```python
from build123d import *

# Parameters (mm, degrees)
SKETCH2_R           = 2.65
BOSS_EXTRUDE1_DEPTH = 10
SKETCH5_R           = 2.5
CHAMFER1_SIZE       = 3
FILLET4_R           = 4
SKETCH9_R           = 6
SKETCH9_R_2         = 2.2
BOSS_EXTRUDE2_DEPTH = 4
LPATTERN1_COUNT     = 2
LPATTERN1_PITCH     = 30
CHAMFER2_SIZE       = 4


with BuildPart() as part:
    # Sketch2 → Boss-Extrude1 (new, symmetric)
    with BuildSketch(Plane.XY):
        with BuildLine():
            ThreePointArc((-73.989796594, 16), (-75.457580373, 6.053392794), (-75.594245813, -4))
            Line((-75.594245813, -4), (-51.34428877, -4))
            ThreePointArc((-51.34428877, -4), (-42.918193786, -7.205281597), (-37.5, 0))
            Line((-37.5, 0), (-21.763957799, 0))
            Line((-21.763957799, 0), (-5.763957799, 16))
            Line((-5.763957799, 16), (-73.989796594, 16))
        make_face()
        with Locations((-45, 0)):
            Circle(SKETCH2_R, mode=Mode.SUBTRACT)
    extrude(amount=BOSS_EXTRUDE1_DEPTH, both=True)

    # Sketch3 → Cut-Revolve1 (revolve, cut)
    with BuildSketch(Plane.XY, mode=Mode.PRIVATE) as cut_revolve1_sk:
        Polygon((-76.457580373, 8), (-75.457580373, 8), (-50.457580373, 8), (-50.457580373, 12.2), (-70.457580373, 12.2), (-76.457580373, 12.2), align=None)
        Polygon((-76.457580373, 15.2), (-76.457580373, 12.2), (-70.457580373, 12.2), align=None)
    revolve(cut_revolve1_sk.sketch.rotate(Axis((-75.457580373, 8, 0), (1, 0, 0)), 90), axis=Axis((-75.457580373, 8, 0), (1, 0, 0)), mode=Mode.SUBTRACT)

    # Cut-Sweep2: sweep along a path in Sketch7
    with BuildLine(Plane.XY) as cut_sweep2_path:
        Line((-50.457580373, 8), (-25.763957799, 8))
        ThreePointArc((-25.763957799, 8), (-22.228423893, 9.464466094), (-20.763957799, 13))
        Line((-20.763957799, 13), (-20.763957799, 16))
    # Sketch5 → Cut-Sweep2 (sweep, cut)
    with BuildSketch(Plane(origin=(0, 16, 0), x_dir=(1, 0, 0), z_dir=(0, 1, 0))):
        with Locations((-20.763957799, 0)):
            Circle(SKETCH5_R)
    sweep(path=cut_sweep2_path.line, mode=Mode.SUBTRACT)

    # Chamfer1
    # the kernel refuses this chamfer: 3 mm, written as the material it takes off along each edge
    with BuildSketch(Plane(origin=(-50.457580373, 8, 0), x_dir=(0, -1, 0), z_dir=(0, 0, 1))) as chamfer1_piece_1_section:
        Polygon((2.5 + CHAMFER1_SIZE, 0), (2.5, CHAMFER1_SIZE), (2.5, 0), align=None)
    chamfer1_piece_1 = revolve(axis=Axis((-50.457580373, 8, 0), (1, 0, 0)), mode=Mode.PRIVATE)
    chamfer1_piece_1 = chamfer1_piece_1 & Plane(origin=(-48.295596493, 8, 0), x_dir=(0, 0, 1), z_dir=(-1, 0, 0)) * Cylinder(4.2, 22, mode=Mode.PRIVATE)
    add(chamfer1_piece_1, mode=Mode.SUBTRACT)

    # Fillet4
    fillet4_edges = [part.edges().sort_by_distance(p)[0] for p in [
        (-21.763957799, 0, 0),
        (-37.5, 0, 0),
        (-51.34428877, -4, 0),
    ]]
    fillet(fillet4_edges, radius=FILLET4_R)

    # Sketch9 → Boss-Extrude2 (add)
    # profile 1 of 3: a face of its own
    with BuildSketch(Plane(origin=(0, 16, 0), x_dir=(1, 0, 0), z_dir=(0, 1, 0))):
        with Locations((-53.989796594, 16)):
            Circle(SKETCH9_R)
        with Locations(Location((-53.989796594, 16, 0), (0, 0, 270))):
            Circle(SKETCH9_R_2, mode=Mode.SUBTRACT)
    # profile 2 of 3: a face of its own
    with BuildSketch(Plane(origin=(0, 16, 0), x_dir=(1, 0, 0), z_dir=(0, 1, 0))):
        with BuildLine():
            ThreePointArc((-47.989796594, 16), (-49.747155907, 11.757359313), (-53.989796594, 10))
            Line((-53.989796594, 10), (-43.989796594, 10))
            Line((-43.989796594, 10), (-48.695678947, 18.823529412))
            ThreePointArc((-48.695678947, 18.823529412), (-48.168941593, 17.45521375), (-47.989796594, 16))
        make_face()
    # profile 3 of 3: a face of its own
    with BuildSketch(Plane(origin=(0, 16, 0), x_dir=(1, 0, 0), z_dir=(0, 1, 0))):
        with BuildLine():
            Line((-59.283914241, 18.823529412), (-63.989796594, 10))
            Line((-63.989796594, 10), (-53.989796594, 10))
            ThreePointArc((-53.989796594, 10), (-59.134754148, 12.913025467), (-59.283914241, 18.823529412))
        make_face()
    boss_extrude2 = extrude(amount=-BOSS_EXTRUDE2_DEPTH)

    # LPattern1: Boss-Extrude2 ×2
    with Locations(*[(i * LPATTERN1_PITCH, 0, 0) for i in range(1, LPATTERN1_COUNT)]):
        add(boss_extrude2)

    # Chamfer2
    # the kernel refuses this chamfer: 4 mm, written as the material it adds along each edge
    with BuildSketch(Plane(origin=(-33.703064642, 12, -10), x_dir=(0, -0.9996219169112968, 0.027495876610586494), z_dir=(-1, 0, 0))) as chamfer2_piece_1_section:
        Polygon((CHAMFER2_SIZE * 0.999621916911, -CHAMFER2_SIZE * 0.0274958766106), (-CHAMFER2_SIZE * 0.0274958766106, -CHAMFER2_SIZE * 0.999621916911), (0, 0), align=None)
    chamfer2_piece_1 = extrude(amount=40.573463904, mode=Mode.PRIVATE)
    chamfer2_piece_1 = split(chamfer2_piece_1, bisect_by=Plane(origin=(-33.908180605, 9.955648468, -10.153029979), z_dir=(0.882352941176471, 0, 0.4705882352941171)), keep=Keep.TOP, mode=Mode.PRIVATE)
    add(chamfer2_piece_1)
    with BuildSketch(Plane(origin=(-33.703064642, 12, -10), x_dir=(0, -0.9996219169112968, 0.027495876610586494), z_dir=(-1, 0, 0))) as chamfer2_piece_2_section:
        Polygon((CHAMFER2_SIZE * 0.999621916911, -CHAMFER2_SIZE * 0.0274958766106), (-CHAMFER2_SIZE * 0.0274958766106, -CHAMFER2_SIZE * 0.999621916911), (0, 0), align=None)
    chamfer2_piece_2 = extrude(amount=40.573463904, mode=Mode.PRIVATE)
    chamfer2_piece_2 = split(chamfer2_piece_2, bisect_by=Plane(origin=(-61.252355545, 10.648848957, -15.132701966), z_dir=(0.882352941176471, 0, 0.4705882352941171)), keep=Keep.TOP, mode=Mode.PRIVATE)
    chamfer2_piece_2 = split(chamfer2_piece_2, bisect_by=Plane(origin=(-46.727237643, 10.648848957, -15.132701966), z_dir=(-0.8823529411764707, 0, 0.4705882352941174)), keep=Keep.TOP, mode=Mode.PRIVATE)
    chamfer2_piece_2 = chamfer2_piece_2 - Plane(origin=(-53.989796594, 10.648848957, -16), x_dir=(0, 0, 1), z_dir=(0, 1, 0)) * Cylinder(2.2, 98, mode=Mode.PRIVATE)
    add(chamfer2_piece_2)
    with BuildSketch(Plane(origin=(-3.703064642, 12, -10), x_dir=(0, -0.9996219169112968, 0.027495876610586494), z_dir=(-1, 0, 0))) as chamfer2_piece_3_section:
        Polygon((CHAMFER2_SIZE * 0.999621916911, -CHAMFER2_SIZE * 0.0274958766106), (-CHAMFER2_SIZE * 0.0274958766106, -CHAMFER2_SIZE * 0.999621916911), (0, 0), align=None)
    chamfer2_piece_3 = extrude(amount=40.573463904, mode=Mode.PRIVATE)
    chamfer2_piece_3 = split(chamfer2_piece_3, bisect_by=Plane(origin=(-31.252355545, 10.648848957, -15.132701966), z_dir=(0.882352941176471, 0, 0.4705882352941171)), keep=Keep.TOP, mode=Mode.PRIVATE)
    chamfer2_piece_3 = split(chamfer2_piece_3, bisect_by=Plane(origin=(-16.727237643, 10.648848957, -15.132701966), z_dir=(-0.8823529411764707, 0, 0.4705882352941174)), keep=Keep.TOP, mode=Mode.PRIVATE)
    chamfer2_piece_3 = chamfer2_piece_3 - Plane(origin=(-23.989796594, 10.648848957, -16), x_dir=(0, 0, 1), z_dir=(0, 1, 0)) * Cylinder(2.2, 98, mode=Mode.PRIVATE)
    add(chamfer2_piece_3)
    with BuildSketch(Plane(origin=(-3.703064642, 12, -10), x_dir=(0, -0.9996219169112968, 0.027495876610586494), z_dir=(-1, 0, 0))) as chamfer2_piece_4_section:
        Polygon((CHAMFER2_SIZE * 0.999621916911, -CHAMFER2_SIZE * 0.0274958766106), (-CHAMFER2_SIZE * 0.0274958766106, -CHAMFER2_SIZE * 0.999621916911), (0, 0), align=None)
    chamfer2_piece_4 = extrude(amount=40.573463904, mode=Mode.PRIVATE)
    chamfer2_piece_4 = split(chamfer2_piece_4, bisect_by=Plane(origin=(-44.071412583, 9.955648468, -10.153029979), z_dir=(-0.8823529411764707, 0, 0.4705882352941174)), keep=Keep.TOP, mode=Mode.PRIVATE)
    add(chamfer2_piece_4)


solid = part.part
```
Geometry: final body of the model. Coordinates: model frame, mm. A direction names the side the tool comes from. Round coordinates to 2 decimals unless told otherwise and drop trailing zeros. Write each loop counter-clockwise with the first axis right and the second up, starting at its lowest first coordinate (ties: lowest second). Pieces come first, ordered by that corner, then holes.
Item 1: Pin query (flat end, axial travel): P1, Ø6, axis at x = -62, y = 13.5, coming from the -Z side; P2, Ø4, axis at x = -50.5, z = -18.5, coming from the -Y side; P3, Ø2, axis at y = -4, z = -0.5, coming from the +X side. Return the tip coordinate at first contact, or that it passes through.
Item 2: Mould query, pull axis X, two halves, no side actions, for faces 4 (the face through (-65, -4, 0)), 5 (the face through (-54, 14, -22)), 6 (the face through (-13.282, 8.482, 0.14)). Classes: +X half, -X half, draft (parallel to the pull), parting line (faces both ways), or undercut.
Item 3: Section query D-D (z = -15). Return loops of the section in (x, y).
Item 4: Material intervals for L1, parallel to Z at x = -65.5, y = 8; L2, parallel to Y at x = -45, z = -4.5; L3, parallel to Y at x = -57.5, z = -12, sorted ascending.
Item 5: Section query A-A (x = -45). Return loops of the section in (y, z), plus the area to 3 significant figures.
Item 6: Section query B-B (z = -9). Return loops of the section in (x, y), plus the area to 3 significant figures.
Item 7: Set-up query: faces 1 (the face through (-36.5, 10.5, -0.1)), 2 (the face through (-24, 12, -19)), 3 (the face through (-19.61, 14.521, 2.218)). Return all of +Z, -Z, +X, -X, +Y, -Y with unobstructed straight access to the full face (end or side cutting, diameter ignored); none if empty.
Item 8: Section query C-C (z = 0). Return loops of the section in (x, y), plus the area to 3 significant figures.
Completed:
1. P1: stops at z = -19.3
1. P2: stops at y = 12
1. P3: stops at x = -38.13
2. face 4: draft
2. face 5: undercut
2. face 6: +X half
3. outline: (-61.32, 12) - (-55.95, 12) - (-55.95, 16) - (-61.32, 16) - close; (-52.03, 12) - (-46.66, 12) - (-46.66, 16) - (-52.03, 16) - close; (-31.32, 12) - (-25.95, 12) - (-25.95, 16) - (-31.32, 16) - close; (-22.03, 12) - (-16.66, 12) - (-16.66, 16) - (-22.03, 16) - close
4. L1: z = -10 to -4.2, 4.2 to 10
4. L2: y = -7.5 to -2.65, 2.65 to 16
4. L3: y = 10 to 16
5. outline: (-7.5, -10) - (-2.65, -10) - (-2.65, 10) - (-7.5, 10) - close; (2.65, -10) - (8, -10) - (9.89, -11.89) - (16, -11.89) - (16, 10) - (2.65, 10) - close; hole circle Ø5 at (8, 0)
5. area: 358 mm2
6. outline: (-75.59, -4) - (-53.26, -4) arc R4 cw to (-50.39, -5.22) arc R7.5 ccw to (-37.97, -2.61) arc R4 cw to (-34.22, 0) - (-23.42, 0) arc R4 ccw to (-20.59, 1.17) - (-5.76, 16) - (-73.99, 16) arc R75.7 ccw to start; hole circle Ø5.3 at (-45, 0)
6. area: 1,140 mm2
7. face 1: -X
7. face 2: -Z, +X, -X, -Y
7. face 3: +Y
8. outline: (-75.69, 1.18) arc R75.7 ccw to (-75.59, -4) - (-53.26, -4) arc R4 cw to (-50.39, -5.22) arc R7.5 ccw to (-37.97, -2.61) arc R4 cw to (-34.22, 0) - (-23.42, 0) arc R4 ccw to (-20.59, 1.17) - (-5.76, 16) - (-18.26, 16) - (-18.26, 13) arc R7.5 cw to (-25.76, 5.5) - (-47.46, 5.5) - (-49.16, 3.8) - (-70.46, 3.8) - close; (-74.37, 14.15) - (-70.46, 12.2) - (-49.16, 12.2) - (-47.46, 10.5) - (-25.76, 10.5) arc R2.5 ccw to (-23.26, 13) - (-23.26, 16) - (-73.99, 16) arc R75.7 ccw to start; hole circle Ø5.3 at (-45, 0)
8. area: 740 mm2
